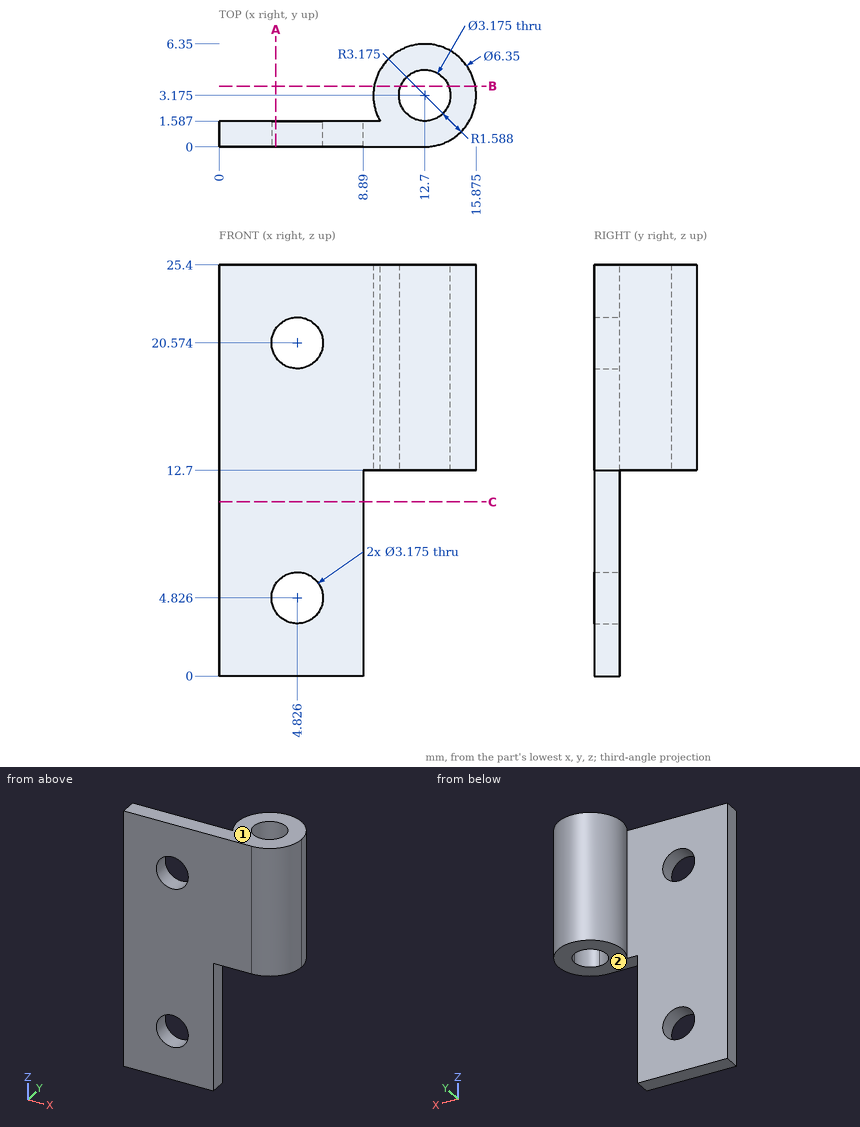
Print and shaded views of the part. All mm, measured from the part's lowest x, y and z. A direction names the side the tool comes from. Coordinates: 2 decimals unless noted, no trailing zeros. Loops run counter-clockwise (first coordinate to the right, second up) from the corner with the lowest first, then second, coordinate; pieces in that order, holes last. Notation, with made-up numbers: (89.5, 72) - (115.5, 72) arc R38 cw to (115.5, 110) - close; hole circle Ø4 at (19, 31). An arc over 180 degrees is marked (long way). Use one line per item in the form item = value. Start each with the question number.
1) Band-saw the part on C-C (z = 10.75). Give the cut face in (x, y).
2) Drill centre lines: L1, parallel to Y at x = 7.75, z = 13.75; L2, parallel to Z at x = 6.25, y = 0.5 (1 decimal); L3, parallel to X at y = 1.75, z = 15.25 (1 decimal). Where is each one in solid material? Low to high. Write a range as from..to.
3) Band-saw the part on A-A (x = 3.5). Give the cut face in (y, z).
4) Flat gauge pins, fed straight in: pin 1 (8 mm diameter, centred on x = 4.5, z = 18.5, fed in from +Y); pin 2 (3 mm diameter, centred on x = 12.7, y = 3.175, fed in from +Z); pin 3 (1.7 mm diameter, centred on y = 0.5, z = 6, fed in from +X); pin 4 (1.5 mm diameter, centred on x = 2, y = 1, fed in from -Z). Where does each tip first touch, or does it go through?
5) Band-saw the part on B-B (y = 3.75). Give the cut face in (x, z).
6) Tool access for the marked faces 1 and 2: list every direction of +Z, -Z, +X, -X, +Y, -Y with a clear straight run to the whole face (end or side of a thin tool).
Check values:
q1.outline = (0, 0) - (8.89, 0) - (8.89, 1.59) - (0, 1.59) - close
q2.L1 = 0..1.59
q2.L2 = 0..4.1, 5.5..19.9, 21.3..25.4
q2.L3 = 9.9..12, 13.4..15.5
q3.outline = (0, 0) - (1.59, 0) - (1.59, 3.95) - (0, 3.95) - close; (0, 5.7) - (1.59, 5.7) - (1.59, 19.7) - (0, 19.7) - close; (0, 21.45) - (1.59, 21.45) - (1.59, 25.4) - (0, 25.4) - close
q4.pin_1 = 1.59
q4.pin_2 = through
q4.pin_3 = 8.89
q4.pin_4 = 0
q5.outline = (9.58, 12.7) - (11.22, 12.7) - (11.22, 25.4) - (9.58, 25.4) - close; (14.18, 12.7) - (15.82, 12.7) - (15.82, 25.4) - (14.18, 25.4) - close
q6.face_1 = +Z, +X, -X, +Y, -Y
q6.face_2 = -Z, +X, +Y, -Y
